Work out the finished part from the listing and answer in its coordinate system (mm). A direction names the side the tool comes from. Coordinates: 2 decimals unless noted, no trailing zeros. Loops run counter-clockwise (first coordinate to the right, second up) from the corner with the lowest first, then second, coordinate; pieces in that order, holes last. Notation, with made-up numbers: (86, -33.75) -> (132, -33.75) arc R25 cw to (132, -17.75) -> close; hole circle Ø2 at (82.5, 35). An arc over 180 degrees is marked (long way). Use a Markdown table: item, result.
from build123d import *

# Parameters (mm, degrees)
EXTRUDE_1_DEPTH     = 30
SKETCH_2_R          = 5
CUT_EXTRUDE_1_DEPTH = 335
SKETCH_3_W          = 30
SKETCH_3_H          = 30
EXTRUDE_2_DEPTH     = 10


with BuildPart() as part:
    # 草圖1 → 填料-伸長1 (new body)
    with BuildSketch(Plane(origin=(0, 0, 0), x_dir=(1, 0, 0), z_dir=(0, 1, 0))):
        Polygon((-100, -150), (100, -150), (100, 150), (15, 150), (15, 50), (-15, 50), (-15, 150), (-100, 150), align=None)
    extrude(amount=EXTRUDE_1_DEPTH)

    # 草圖2 → 除料-伸長1 (cut)
    with BuildSketch(Plane.ZY.offset(100)):
        with Locations((-100, 15)):
            Circle(SKETCH_2_R)
        with Locations((110, 15)):
            Circle(SKETCH_2_R)
    extrude(amount=-CUT_EXTRUDE_1_DEPTH, mode=Mode.SUBTRACT)

    # 草圖3 → 填料-伸長2 (add)
    with BuildSketch(Plane(origin=(0, 30, 0), x_dir=(1, 0, 0), z_dir=(0, 1, 0))):
        Rectangle(SKETCH_3_W, SKETCH_3_H)
    extrude(amount=EXTRUDE_2_DEPTH)


solid = part.part
Q1. Consider line 1 (Y direction, x = 71, z = -100); line 2 (X direction, y = 27.5, z = -109); line 3 (Z direction, x = -49, y = 10.5). Determine where each line is inside the solid, lowest interval first. Write a range as [from, to].
Solved:
| item | result |
|---|---|
| line 1 | [0, 10], [20, 30] |
| line 2 | [-100, -15], [15, 100] |
| line 3 | [-150, -102.18], [-97.82, 107.82], [112.18, 150] |
Q2. Section D-D on z = -100 is taken. Determine the outline of the cut face in (x, y), and give its area (3 significant figures).
Solved:
| item | result |
|---|---|
| outline | (-100, 0) -> (-15, 0) -> (-15, 10) -> (-100, 10) -> close; (-100, 20) -> (-15, 20) -> (-15, 30) -> (-100, 30) -> close; (15, 0) -> (100, 0) -> (100, 10) -> (15, 10) -> close; (15, 20) -> (100, 20) -> (100, 30) -> (15, 30) -> close |
| area | 3,400 mm² |
Q3. Section A-A on z = 110 is taken. Determine the outline of the cut face in (x, y).
Solved:
| item | result |
|---|---|
| outline | (-100, 0) -> (100, 0) -> (100, 10) -> (-100, 10) -> close; (-100, 20) -> (100, 20) -> (100, 30) -> (-100, 30) -> close |
Q4. Section B-B on y = 15 is taken. Determine the outline of the cut face in (x, z).
Solved:
| item | result |
|---|---|
| outline | (-100, -150) -> (-15, -150) -> (-15, -105) -> (-100, -105) -> close; (-100, -95) -> (-15, -95) -> (-15, -50) -> (15, -50) -> (15, -95) -> (100, -95) -> (100, 105) -> (-100, 105) -> close; (-100, 115) -> (100, 115) -> (100, 150) -> (-100, 150) -> close; (15, -150) -> (100, -150) -> (100, -105) -> (15, -105) -> close |
Q5. Section C-C on x = 67.5 is taken. Determine the outline of the cut face in (y, z), and give its area (3 significant figures).
Solved:
| item | result |
|---|---|
| outline | (0, -150) -> (30, -150) -> (30, 150) -> (0, 150) -> close; hole circle Ø10 at (15, -100); hole circle Ø10 at (15, 110) |
| area | 8,840 mm² |
Q6. Given pin 1 Ø1.5 at (y, z) = (36, 11) entering from +X; pin 2 Ø11 at (y, z) = (36, 7) entering from -X; pin 3 Ø3 at (x, y) = (-1, 36.5) entering from +Z, each flat-ended and moving along its own axis, determine where each tip first touches the part or whether it passes through.
Solved:
| item | result |
|---|---|
| pin 1 | x = 15 |
| pin 2 | x = -15 |
| pin 3 | z = 15 |
Q7. Determine the mould class of faces 1 (the flat face through (0, 35, -15)), 2 (the cylindrical face through (56.905, 13.085, -95.381)), 3 (the cylindrical face through (-1.4, 13.085, 114.619)), 4 (the flat face through (-1, 0, -2)) for opening direction Z: pulls with the +Z half, pulls with the -Z half, needs draft (parallel to the pull), parting line crosses it, or undercut.
Solved:
| item | result |
|---|---|
| face 1 | pulls with the -Z half |
| face 2 | undercut |
| face 3 | undercut |
| face 4 | needs draft |
Q8. For faces 5 (the flat face through (0, 35, 15)), 6 (the flat face through (15, 35, 0)), 7 (the flat face through (15, 8, -101)), 8 (the flat face through (-15, 35, 0)), 9 (the flat face through (58, 15, -150)), determine the directions among +Z, -Z, +X, -X, +Y, -Y from which every point of the face is accessible in a straight line to the end or side of a thin tool.
Solved:
| item | result |
|---|---|
| face 5 | +Z, +X, -X, +Y |
| face 6 | +Z, -Z, +X, +Y |
| face 7 | -Z, +Y, -Y |
| face 8 | +Z, -Z, -X, +Y |
| face 9 | -Z, +X, -X, +Y, -Y |
